Build history of the part. All positions in model axes, mm. A direction names the side the tool comes from. Round coordinates to 2 decimals unless told otherwise and drop trailing zeros. Write each loop counter-clockwise with the first axis right and the second up, starting at its lowest first coordinate (ties: lowest second). Pieces come first, ordered by that corner, then holes. Notation, with made-up numbers: (-38, -39) -> (-12, -39) arc R29 ccw to (-12, -1) -> close; hole circle Ø6 at (76.5, -18). An arc over 180 degrees is marked (long way). Return JSON: item names as keys, results as strings.
from build123d import *

# Parameters (mm, degrees)
F0_W         = 20.32
F0_H         = 50.8
F1_DEPTH     = 12.7
F2_W         = 15.24
F2_H         = 45.72
F3_DEPTH     = 5.08
F4_W         = 3.2004
F4_H         = 3.5052
F5_DEPTH     = 2.54
F6_W         = 5.08
F6_H         = 7.62
F7_DEPTH     = 25.4
F8_T1_DEPTH  = 76.2
F8_T3_DEPTH  = 45.72
F8_T5_DEPTH  = 7.62
F8_T7_DEPTH  = 5.08
F8_T13_DEPTH = 20.32
F8_T17_DEPTH = 17.78
F8_T24_DEPTH = 20.32
F8_T28_DEPTH = 17.78
F8_T35_DEPTH = 17.78
F8_T39_DEPTH = 20.32
F8_T46_DEPTH = 20.32
F8_T50_DEPTH = 17.78
F9_R         = 0.635
F10_DEPTH    = 25.4


# Not quite as in the source:
# - a fillet or chamfer that OpenCascade refuses, or shapes differently, is made with other operations: its cross-section is extruded or revolved along the edge and cut away or added


with BuildPart() as f1:
    # F0 (on Top) → F1 (new body)
    with BuildSketch(Plane.XY):
        Rectangle(F0_W, F0_H)
    extrude(amount=F1_DEPTH)

    # F2 (on Top) → F3 (cut)
    with BuildSketch(Plane.XY):
        Rectangle(F2_W, F2_H)
    extrude(amount=F3_DEPTH, mode=Mode.SUBTRACT)

    # F4 (on face) → F5 (cut)
    with BuildSketch(Plane(origin=(0, 0, 5.08), x_dir=(1, 0, 0), z_dir=(0, 0, -1))):
        with Locations((0, -20.5359)):
            Rectangle(F4_W, F4_H)
    extrude(amount=-F5_DEPTH, mode=Mode.SUBTRACT)

    # F6 (on Top) → F7 (cut)
    with BuildSketch(Plane.XY):
        with Locations((0, 13.1445)):
            Rectangle(F6_W, F6_H)
    extrude(amount=F7_DEPTH, mode=Mode.SUBTRACT)

    # F8: fillet of radius 5.08 on 8 edges, made by hand

    # F8_s2 → F8_t1 (cut)
    with BuildSketch(Plane.XZ.offset(-38.1)):
        with BuildLine():
            ThreePointArc((10.16, 7.62), (8.6721024484, 11.2121024484), (5.08, 12.7))
            Line((5.08, 12.7), (10.16, 12.7))
            Line((10.16, 12.7), (10.16, 7.62))
        make_face()
        with BuildLine():
            ThreePointArc((-5.08, 12.7), (-8.6721024484, 11.2121024484), (-10.16, 7.62))
            Line((-10.16, 7.62), (-10.16, 12.7))
            Line((-10.16, 12.7), (-5.08, 12.7))
        make_face()
    extrude(amount=F8_T1_DEPTH, mode=Mode.SUBTRACT)

    # F8_s4 → F8_t3 (cut)
    with BuildSketch(Plane.YZ.offset(-22.86)):
        with BuildLine():
            ThreePointArc((-25.4, 7.62), (-23.9121024484, 11.2121024484), (-20.32, 12.7))
            Line((-20.32, 12.7), (-25.4, 12.7))
            Line((-25.4, 12.7), (-25.4, 7.62))
        make_face()
        with BuildLine():
            ThreePointArc((25.4, 7.62), (23.9121024484, 11.2121024484), (20.32, 12.7))
            Line((20.32, 12.7), (25.4, 12.7))
            Line((25.4, 12.7), (25.4, 7.62))
        make_face()
    extrude(amount=F8_T3_DEPTH, mode=Mode.SUBTRACT)

    # F8_s6 → F8_t5 (cut)
    with BuildSketch(Plane.XZ.offset(-16.9545)):
        with BuildLine():
            ThreePointArc((7.62, 12.7), (4.0278975516, 11.2121024484), (2.54, 7.62))
            Line((2.54, 7.62), (2.54, 12.7))
            Line((2.54, 12.7), (7.62, 12.7))
        make_face()
        with BuildLine():
            ThreePointArc((-7.62, 12.7), (-4.0278975516, 11.2121024484), (-2.54, 7.62))
            Line((-2.54, 7.62), (-2.54, 12.7))
            Line((-2.54, 12.7), (-7.62, 12.7))
        make_face()
    extrude(amount=F8_T5_DEPTH, mode=Mode.SUBTRACT)

    # F8_s8 → F8_t7 (cut)
    with BuildSketch(Plane.YZ.offset(-2.54)):
        with BuildLine():
            ThreePointArc((22.0345, 12.7), (18.4423975516, 11.2121024484), (16.9545, 7.62))
            Line((16.9545, 7.62), (16.9545, 12.7))
            Line((16.9545, 12.7), (22.0345, 12.7))
        make_face()
        with BuildLine():
            ThreePointArc((4.2545, 12.7), (7.8466024484, 11.2121024484), (9.3345, 7.62))
            Line((9.3345, 7.62), (9.3345, 12.7))
            Line((9.3345, 12.7), (4.2545, 12.7))
        make_face()
    extrude(amount=F8_T7_DEPTH, mode=Mode.SUBTRACT)


with BuildPart() as f8_tool11:
    # F8_s12 → F8_t13 (new body)
    with BuildSketch(Plane.XZ.offset(-29.6545)):
        with BuildLine():
            ThreePointArc((7.62, 12.7), (4.0278975516, 11.2121024484), (2.54, 7.62))
            Line((2.54, 7.62), (2.54, 12.7))
            Line((2.54, 12.7), (7.62, 12.7))
        make_face()
    extrude(amount=F8_T13_DEPTH)

    split(bisect_by=Plane.XZ.offset(-16.9545), keep=Keep.BOTTOM)


with BuildPart() as f8_tool15:
    # F8_s16 → F8_t17 (new body)
    with BuildSketch(Plane.YZ.offset(-2.54)):
        with BuildLine():
            ThreePointArc((22.0345, 12.7), (18.4423975516, 11.2121024484), (16.9545, 7.62))
            Line((16.9545, 7.62), (16.9545, 12.7))
            Line((16.9545, 12.7), (22.0345, 12.7))
        make_face()
    extrude(amount=F8_T17_DEPTH)

    split(bisect_by=Plane.YZ.offset(2.54), keep=Keep.TOP)


with BuildPart() as f8_tool11_1:
    add(f8_tool11.part)

    # F8_t19: intersect F8_tool15
    add(f8_tool15.part, mode=Mode.INTERSECT)


with BuildPart() as f1_1:
    add(f1.part)

    # F8_t9: cut F8_tool11
    add(f8_tool11_1.part, mode=Mode.SUBTRACT)


with BuildPart() as f8_tool22:
    # F8_s23 → F8_t24 (new body)
    with BuildSketch(Plane.XZ.offset(-16.9545)):
        with BuildLine():
            ThreePointArc((7.62, 12.7), (4.0278975516, 11.2121024484), (2.54, 7.62))
            Line((2.54, 7.62), (2.54, 12.7))
            Line((2.54, 12.7), (7.62, 12.7))
        make_face()
    extrude(amount=F8_T24_DEPTH)

    split(bisect_by=Plane.XZ.offset(-9.3345), keep=Keep.TOP)


with BuildPart() as f8_tool26:
    # F8_s27 → F8_t28 (new body)
    with BuildSketch(Plane.YZ.offset(15.24)):
        with BuildLine():
            ThreePointArc((4.2545, 12.7), (7.8466024484, 11.2121024484), (9.3345, 7.62))
            Line((9.3345, 7.62), (9.3345, 12.7))
            Line((9.3345, 12.7), (4.2545, 12.7))
        make_face()
    extrude(amount=-F8_T28_DEPTH)

    split(bisect_by=Plane.YZ.offset(2.54), keep=Keep.TOP)


with BuildPart() as f8_tool22_1:
    add(f8_tool22.part)

    # F8_t30: intersect F8_tool26
    add(f8_tool26.part, mode=Mode.INTERSECT)


with BuildPart() as f1_2:
    add(f1_1.part)

    # F8_t20: cut F8_tool22
    add(f8_tool22_1.part, mode=Mode.SUBTRACT)


with BuildPart() as f8_tool33:
    # F8_s34 → F8_t35 (new body)
    with BuildSketch(Plane.YZ.offset(-15.24)):
        with BuildLine():
            ThreePointArc((22.0345, 12.7), (18.4423975516, 11.2121024484), (16.9545, 7.62))
            Line((16.9545, 7.62), (16.9545, 12.7))
            Line((16.9545, 12.7), (22.0345, 12.7))
        make_face()
    extrude(amount=F8_T35_DEPTH)

    split(bisect_by=Plane.YZ.offset(-2.54), keep=Keep.BOTTOM)


with BuildPart() as f8_tool37:
    # F8_s38 → F8_t39 (new body)
    with BuildSketch(Plane.XZ.offset(-9.3345)):
        with BuildLine():
            ThreePointArc((-7.62, 12.7), (-4.0278975516, 11.2121024484), (-2.54, 7.62))
            Line((-2.54, 7.62), (-2.54, 12.7))
            Line((-2.54, 12.7), (-7.62, 12.7))
        make_face()
    extrude(amount=-F8_T39_DEPTH)

    split(bisect_by=Plane.XZ.offset(-16.9545), keep=Keep.BOTTOM)


with BuildPart() as f8_tool33_1:
    add(f8_tool33.part)

    # F8_t41: intersect F8_tool37
    add(f8_tool37.part, mode=Mode.INTERSECT)


with BuildPart() as f1_3:
    add(f1_2.part)

    # F8_t31: cut F8_tool33
    add(f8_tool33_1.part, mode=Mode.SUBTRACT)


with BuildPart() as f8_tool44:
    # F8_s45 → F8_t46 (new body)
    with BuildSketch(Plane.XZ.offset(3.3655)):
        with BuildLine():
            ThreePointArc((-7.62, 12.7), (-4.0278975516, 11.2121024484), (-2.54, 7.62))
            Line((-2.54, 7.62), (-2.54, 12.7))
            Line((-2.54, 12.7), (-7.62, 12.7))
        make_face()
    extrude(amount=-F8_T46_DEPTH)

    split(bisect_by=Plane.XZ.offset(-9.3345), keep=Keep.TOP)


with BuildPart() as f8_tool48:
    # F8_s49 → F8_t50 (new body)
    with BuildSketch(Plane.YZ.offset(2.54)):
        with BuildLine():
            ThreePointArc((4.2545, 12.7), (7.8466024484, 11.2121024484), (9.3345, 7.62))
            Line((9.3345, 7.62), (9.3345, 12.7))
            Line((9.3345, 12.7), (4.2545, 12.7))
        make_face()
    extrude(amount=-F8_T50_DEPTH)

    split(bisect_by=Plane.YZ.offset(-2.54), keep=Keep.BOTTOM)


with BuildPart() as f8_tool44_1:
    add(f8_tool44.part)

    # F8_t52: intersect F8_tool48
    add(f8_tool48.part, mode=Mode.INTERSECT)


with BuildPart() as f1_4:
    add(f1_3.part)

    # F8_t42: cut F8_tool44
    add(f8_tool44_1.part, mode=Mode.SUBTRACT)

    # F9 (on face) → F10 (cut)
    with BuildSketch(Plane(origin=(0, 0, 7.62), x_dir=(1, 0, 0), z_dir=(0, 0, -1))):
        with Locations((0, -20.460145548)):
            Circle(F9_R)
    extrude(amount=-F10_DEPTH, mode=Mode.SUBTRACT)


solid = f1_4.part
Q1. Wall check: L1, parallel to Y at x = 1.25, z = 5.25; L2, parallel to Y at x = 0, z = 10.8; L3, parallel to X at y = 11.5, z = 5.75. Give the ranges that are in metal, low to high.
Verdict:
{"L1": "y = -25.4 to 9.33, 16.95 to 18.78, 22.29 to 25.4", "L2": "y = -24.28 to 8.22, 18.07 to 19.83, 21.1 to 24.28", "L3": "x = -10.16 to -2.54, 2.54 to 10.16"}
Q2. Saw through at A-A on z = 3.5. List the corners of the cut face in (x, y), then the cut area to 3 significant figures.
Verdict:
{"outline": "(-10.16, -25.4) -> (10.16, -25.4) -> (10.16, 25.4) -> (-10.16, 25.4) -> close; hole (-7.62, -22.86) -> (7.62, -22.86) -> (7.62, 22.86) -> (-7.62, 22.86) -> close", "area": "335 mm²"}
Q3. Saw through at C-C on y = 16. List the corners of the cut face in (x, z).
Verdict:
{"outline": "(-10.16, 0) -> (-7.62, 0) -> (-7.62, 5.08) -> (-2.54, 5.08) -> (-2.54, 7.62) arc R5.08 ccw to (-6.35, 12.54) arc R5.08 ccw to (-10.16, 7.62) -> close; (2.54, 5.08) -> (7.62, 5.08) -> (7.62, 0) -> (10.16, 0) -> (10.16, 7.62) arc R5.08 ccw to (6.35, 12.54) arc R5.08 ccw to (2.54, 7.62) -> close"}
Q4. Pin check, flat tips, straight feed: pin 1 Ø1 at (x, y) = (0, 20) entering from -Z; pin 2 Ø4.5 at (x, y) = (0.5, -3.5) entering from -Z. Stop position of each tip, or through.
Verdict:
{"pin 1": "stops at z = 7.62", "pin 2": "stops at z = 5.08"}
Q5. 3-axis set-ups, long thin cutter, end or side, ignore diameter. For faces 4 (the cylindrical face through (0.089, 7.122, 11.813)), 5 (the flat face through (-1.6, 21, 6)), 6 (the cylindrical face through (-0.1, 24.2, 10.9)): which of +Z, -Z, +X, -X, +Y, -Y reach the whole face in a straight line?
Verdict:
{"face 4": "+Z", "face 5": "-Z", "face 6": "+Z, +X, -X, +Y"}
Q6. Saw through at B-B on x = 0. List the corners of the cut face in (y, z).
Verdict:
{"outline": "(-25.4, 0) -> (-22.86, 0) -> (-22.86, 5.08) -> (9.33, 5.08) -> (9.33, 7.62) arc R5.08 ccw to (4.25, 12.7) -> (-20.32, 12.7) arc R5.08 ccw to (-25.4, 7.62) -> close; (16.95, 5.08) -> (18.78, 5.08) -> (18.78, 7.62) -> (19.83, 7.62) -> (19.83, 12.19) arc R5.08 ccw to (16.95, 7.62) -> close; (21.1, 7.62) -> (22.29, 7.62) -> (22.29, 5.08) -> (22.86, 5.08) -> (22.86, 0) -> (25.4, 0) -> (25.4, 7.62) arc R5.08 ccw to (21.18, 12.63) arc R5.08 ccw to (21.1, 12.61) -> close"}
Q7. Saw through at D-D on y = -16.5. List the corners of the cut face in (x, z), then the cut area to 3 significant figures.
Verdict:
{"outline": "(-10.16, 0) -> (-7.62, 0) -> (-7.62, 5.08) -> (7.62, 5.08) -> (7.62, 0) -> (10.16, 0) -> (10.16, 7.62) arc R5.08 ccw to (5.08, 12.7) -> (-5.08, 12.7) arc R5.08 ccw to (-10.16, 7.62) -> close", "area": "170 mm²"}
Q8. Two-plate mould, pull along Y, no slides. Class faces 1 (the flat face through (0, -25.4, 4)), 2 (the flat face through (0, 25.4, 4)), 3 (the flat face through (0, 18.783, 6)): +Y half, -Y half, draft (parallel to the pull), parting line (faces both ways), or undercut.
Verdict:
{"face 1": "-Y half", "face 2": "+Y half", "face 3": "undercut"}
